from build123d import *

# Parameters (mm, degrees)
F0_R     = 2.942768
F0_R_2   = 3.175
F0_R_3   = 2.610476
F0_R_4   = 4.179488
F1_DEPTH = 3.048


with BuildPart() as f1:
    # F0 (on Front) → F1 (new body)
    with BuildSketch(Plane.XZ):
        with BuildLine():
            ThreePointArc((9.45896, 115.419686), (9.508476, 114.860816), (9.525, 114.3))
            ThreePointArc((9.525, 114.3), (0.351146, 104.781475), (-9.49911, 113.598185))
            Line((-9.49911, 113.598185), (-15.742671, 65.545469))
            ThreePointArc((-15.742671, 65.545469), (-1.643104, 79.289738), (14.984226, 68.742956))
            Line((14.984226, 68.742956), (9.45896, 115.419686))
        make_face()
        with Locations((-4.530268, 100.0252)):
            Circle(F0_R, mode=Mode.SUBTRACT)
        with BuildLine():
            Line((15.794203, 61.90038), (14.984226, 68.742956))
            ThreePointArc((14.984226, 68.742956), (-1.643104, 79.289738), (-15.742671, 65.545469))
            Line((-15.742671, 65.545469), (-15.077269, 58.530939))
            ThreePointArc((-15.077269, 58.530939), (1.722435, 47.718719), (15.794203, 61.90038))
        make_face()
        with Locations((0, 63.5)):
            Circle(F0_R_2, mode=Mode.SUBTRACT)
        with BuildLine():
            Line((11.307223, 17.59718), (15.794203, 61.90038))
            ThreePointArc((15.794203, 61.90038), (1.722435, 47.718719), (-15.077269, 58.530939))
            Line((-15.077269, 58.530939), (-9.525, 0))
            ThreePointArc((-9.525, 0), (0, 9.525), (9.525, 0))
            ThreePointArc((9.525, 0), (6.970557, -6.491299), (0.677344, -9.500886))
            Line((0.677344, -9.500886), (44.732405, -7.932475))
            ThreePointArc((44.732405, -7.932475), (36.5125, 0), (44.732405, 7.932475))
            Line((44.732405, 7.932475), (18.934103, 8.850924))
            ThreePointArc((18.934103, 8.850924), (13.224974, 11.57098), (11.307223, 17.59718))
        make_face()
        with BuildLine():
            ThreePointArc((52.3875, 0), (50.161633, 5.51191), (44.732405, 7.932475))
            ThreePointArc((44.732405, 7.932475), (36.5125, 0), (44.732405, -7.932475))
            ThreePointArc((44.732405, -7.932475), (50.161633, -5.51191), (52.3875, 0))
        make_face()
        with Locations((44.45, 0)):
            Circle(F0_R_3, mode=Mode.SUBTRACT)
        with BuildLine():
            ThreePointArc((9.525, 0), (0, 9.525), (-9.525, 0))
            ThreePointArc((-9.525, 0), (-6.735192, -6.735192), (0, -9.525))
            Line((0, -9.525), (0.677344, -9.500886))
            ThreePointArc((0.677344, -9.500886), (6.970557, -6.491299), (9.525, 0))
        make_face()
        Circle(F0_R_4, mode=Mode.SUBTRACT)
        with BuildLine():
            ThreePointArc((-9.49911, 113.598185), (0.351146, 104.781475), (9.525, 114.3))
            ThreePointArc((9.525, 114.3), (9.508476, 114.860816), (9.45896, 115.419686))
            ThreePointArc((9.45896, 115.419686), (-0.910971, 123.781337), (-9.49911, 113.598185))
        make_face()
        with Locations((0, 114.3)):
            Circle(F0_R_2, mode=Mode.SUBTRACT)
    extrude(amount=-F1_DEPTH)


solid = f1.part
Can you work these out from the model? Positions are in its coordinate system, mm. A direction names the side the tool comes from. Round coordinates to 2 decimals unless told otherwise and drop trailing zeros. Loops run counter-clockwise (first coordinate to the right, second up) from the corner with the lowest first, then second, coordinate; pieces in that order, holes last. Notation, with made-up numbers: (14.5, -11) - (41.5, -11) arc R31 ccw to (41.5, 23) - close; hole circle Ø3 at (20, 15). An arc over 180 degrees is marked (long way). Answer in a Markdown table with one row per item. Add a question column.
Q1. I need wall thicknesses on L1, parallel to X at y = 2.2, z = 1; L2, parallel to Z at x = 44.45, y = 1.2; L3, parallel to Z at x = -2, y = 2. Which ranges of each line are inside material? Lowest first, please.
Q2. I want a section at C-C on x = 23. List the corners of the cut face in (y, z) for me, and give its area (3 significant figures).
Q3. For pin 1 Ø4 at (x, z) = (0, 114.3) entering from -Y; pin 2 Ø1 at (y, z) = (1.5, 100.5) entering from +X; pin 3 Ø1.5 at (y, z) = (2.5, 94.5) entering from +X; pin 4 Ø1.5 at (x, y) = (41.5, 1) entering from -Z, each with a flat end and sliding along its axis, tell me the tip position at first contact or that it passes through.
Q4. We'd pull the mould along Z, two halves only. Please class faces 3 (the cylindrical face through (-6.81, 1.5, -6.66)), 4 (the cylindrical face through (13.29, 1.5, 11.5)), 5 (the flat face through (3, 3.048, 43)): pulls with the +Z half, pulls with the -Z half, needs draft (parallel to the pull), parting line crosses it, or undercut.
Q5. I want a section at A-A on z = 63.5. List the corners of the cut face in (x, y) for me (3 decimals).
Q6. I want a section at B-B on y = 1.4. Count the separate pieces of the cut face and the enclosed holes in it, and give its area (3 significant figures).
Q7. I want a section at D-D on z = 42.5. List the corners of the cut face in (x, y) for me.
Q8. Which directions (+Z, -Z, +X, -X, +Y, -Y) give clear straight access to the entire face, cutting with the end or side of a thin tool? Please do faces 1 (the cylindrical face through (1.707, 1.503, 66.177)), 2 (the flat face through (13.52, 1.5, 39.44)).
A:
| question | item | result |
|---|---|---|
| 1 | L1 | -9.62 to -4.06, 4.06 to 42.04, 46.86 to 52.32 |
| 1 | L2 | -7.94 to -2.61, 2.61 to 7.94 |
| 1 | L3 | -9.31 to -3.67, 3.67 to 61.03, 65.97 to 98.52, 101.53 to 111.83, 116.77 to 123.61 |
| 2 | outline | (0, -8.71) - (3.05, -8.71) - (3.05, 8.71) - (0, 8.71) - close |
| 2 | area | 53.1 mm^2 |
| 3 | pin 1 | through |
| 3 | pin 2 | x = 11.28 |
| 3 | pin 3 | x = 12.02 |
| 3 | pin 4 | z = -8.07 |
| 4 | face 3 | pulls with the -Z half |
| 4 | face 4 | undercut |
| 4 | face 5 | needs draft |
| 5 | outline | (-15.549, 0) - (-3.175, 0) - (-3.175, 3.048) - (-15.549, 3.048) - close; (3.175, 0) - (15.605, 0) - (15.605, 3.048) - (3.175, 3.048) - close |
| 6 | separate pieces | 1 |
| 6 | enclosed holes | 5 |
| 6 | area | 3,730 mm^2 |
| 7 | outline | (-13.56, 0) - (13.83, 0) - (13.83, 3.05) - (-13.56, 3.05) - close |
| 8 | face 1 | +Y, -Y |
| 8 | face 2 | +X, +Y, -Y |
